CAD build for the part. Positions are in the model's coordinates, mm. Face numbers are marked on the shaded views. Give positions to 0.01 mm unless a question says otherwise; leave off trailing zeros. Loops run counter-clockwise (first coordinate to the right, second up) from the corner with the lowest first, then second, coordinate; pieces in that order, holes last.
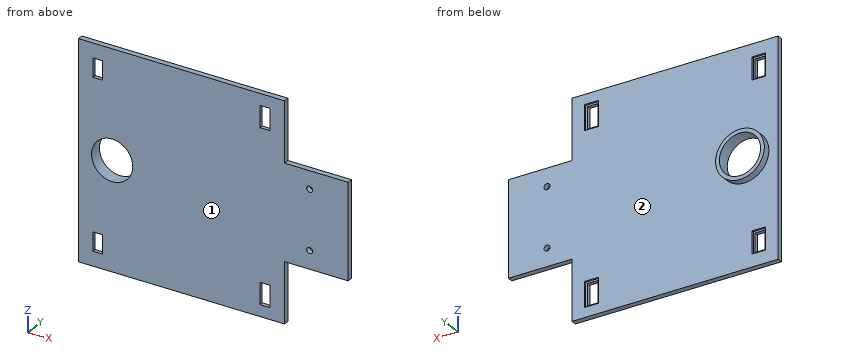
Autodesk Inventor part; units mm, degrees
ref_plane "YZ Plane" through (0, 0, 0) normal (1, 0, 0) x (0, 1, 0)
ref_plane "XZ Plane" through (0, 0, 0) normal (0, 1, 0) x (-1, 0, 0)
ref_plane "XY Plane" through (0, 0, 0) normal (0, 0, 1) x (1, 0, 0)
sketch "Boceto1" plane through (0, 0, 0) normal (0, 1, 0) x (-1, 0, 0)
  line L0 (25.35, 26.5) -> (0, 26.5)
  line L1 (0, 26.5) -> (0, -26.5)
  line L2 (0, -26.5) -> (25.35, -26.5)
  line L3 (-8.9327, 0) -> (109.0416, 0) construction
  line L4 (25.35, 60) -> (150, 60)
  line L5 (150, 60) -> (150, -60)
  line L6 (150, -60) -> (25.35, -60)
  line L7 (25.35, -60) -> (25.35, -26.5)
  line L8 (25.35, 26.5) -> (25.35, 60)
  circle A0 centre (21.45, 16.5) radius 1.65
  circle A1 centre (21.45, -16.5) radius 1.65
  point P0 (0, 0)
  point P1 (0, 0)
  dimension "d1" = 53
  dimension "d2" = 120
  dimension "d3" = 124.65
  dimension "d4" = 25.35
  dimension "d6" = 33.5
  dimension "d8" = 3.3
  dimension "d9" = 16.5
  dimension "d10" = 3.9
extrude "Extrusión1" add sketch "Boceto1" along normal blind 3
sketch "Boceto2" plane through (0, 3, 0) normal (0, 1, 0) x (1, 0, 0)
  line L0 (-150, 60) -> (-150, -60)
  line L1 (-25.35, 60) -> (-150, 60)
  line L2 (-150, -60) -> (-25.35, -60)
  line L3 (-25.35, -60) -> (-25.35, 60)
  line L4 (-25.35, 60) -> (-150, 60)
  line L5 (-150, 60) -> (-150, -60)
  line L6 (-30.35, -55) -> (-145, -55)
  line L7 (-145, -55) -> (-145, 55)
  line L8 (-145, 55) -> (-30.35, 55)
  line L9 (-30.35, 55) -> (-30.35, -55)
  circle A0 centre (-131.25, 0) radius 11.465
  circle A1 centre (-131.25, 0) radius 13.55
  point P0 (0, 0)
  dimension "d13" = 5
  dimension "d14" = 22.93
  dimension "d15" = 13.75
  dimension "d16" = 27.1
extrude "Extrusión2" cut sketch "Boceto2" against normal through all contours A0
extrude "Extrusión3" add sketch "Boceto2" along normal blind 4 contours A1
sketch "Boceto3" plane through (0, 3, 0) normal (0, 1, 0) x (1, 0, 0)
  line L0 (-25.35, 26.5) -> (-25.35, 60)
  line L1 (-25.35, 60) -> (-35.35, 60)
  line L2 (-35.35, 60) -> (-35.35, 26.5)
  line L3 (-35.35, 26.5) -> (-25.35, 26.5)
  line L4 (-25.35, 26.5) -> (-25.35, 60)
  line L5 (-25.35, -60) -> (-25.35, -26.5)
  line L6 (-25.35, -60) -> (-35.35, -60)
  line L7 (-35.35, -60) -> (-35.35, -26.5)
  line L8 (-35.35, -26.5) -> (-25.35, -26.5)
  line L9 (-25.35, -26.5) -> (-25.35, -60)
  point P0 (-150, 60)
  dimension "d46" = 10
  dimension "d47" = 10
  dimension "d48" = 33.5
  dimension "d49" = 33.5
extrude "Extrusión7" cut sketch "Boceto3" against normal through all
sketch "Boceto4" plane through (0, 3, 0) normal (0, 1, 0) x (1, 0, 0)
  line L0 (-143, 53) -> (-135.55, 53)
  line L1 (-135.55, 53) -> (-135.55, 40.55)
  line L2 (-135.55, 40.55) -> (-143, 40.55)
  line L3 (-143, 40.55) -> (-143, 53)
  line L4 (-136.55, 52) -> (-142, 52)
  line L5 (-142, 52) -> (-142, 41.55)
  line L6 (-142, 41.55) -> (-136.55, 41.55)
  line L7 (-136.55, 41.55) -> (-136.55, 52)
  line L8 (-50.1, 54.55) -> (-42.35, 54.55)
  line L9 (-42.35, 54.55) -> (-42.35, 40.55)
  line L10 (-42.35, 40.55) -> (-50.1, 40.55)
  line L11 (-50.1, 40.55) -> (-50.1, 54.55)
  line L12 (-43.35, 53.55) -> (-49.1, 53.55)
  line L13 (-49.1, 53.55) -> (-49.1, 41.55)
  line L14 (-49.1, 41.55) -> (-43.35, 41.55)
  line L15 (-43.35, 41.55) -> (-43.35, 53.55)
  line L16 (-35.35, 60) -> (-150, 60) construction
  line L17 (-35.35, -26.5) -> (-35.35, -60) construction
  line L18 (-150, 60) -> (-35.35, 60) construction
  line L19 (-35.35, 60) -> (-35.35, -60) construction
  line L20 (-35.35, -60) -> (-150, -60) construction
  line L21 (-150, -60) -> (-150, 60) construction
  line L22 (-147, 57) -> (-38.35, 57) construction
  line L23 (-38.35, 57) -> (-38.35, -57) construction
  line L24 (-38.35, -57) -> (-147, -57) construction
  line L25 (-147, -57) -> (-147, 57) construction
  line L26 (-150, 0) -> (0, 0) construction
  line L27 (-50.1, -40.55) -> (-50.1, -54.55)
  line L28 (-136.55, -41.55) -> (-136.55, -52)
  line L29 (-135.55, -53) -> (-135.55, -40.55)
  line L30 (-136.55, -52) -> (-142, -52)
  line L31 (-142, -52) -> (-142, -41.55)
  line L32 (-142, -41.55) -> (-136.55, -41.55)
  line L33 (-143, -53) -> (-135.55, -53)
  line L34 (-135.55, -40.55) -> (-143, -40.55)
  line L35 (-143, -40.55) -> (-143, -53)
  line L36 (-42.35, -40.55) -> (-50.1, -40.55)
  line L37 (-42.35, -54.55) -> (-42.35, -40.55)
  line L38 (-50.1, -54.55) -> (-42.35, -54.55)
  line L39 (-43.35, -53.55) -> (-49.1, -53.55)
  line L40 (-49.1, -53.55) -> (-49.1, -41.55)
  line L41 (-49.1, -41.55) -> (-43.35, -41.55)
  line L42 (-43.35, -41.55) -> (-43.35, -53.55)
  point P0 (-46.225, 40.55)
  point P1 (-139.275, 40.55)
  point P2 (-46.225, -40.55)
  point P3 (-139.275, -40.55)
  dimension "d52" = 7.45
  dimension "d53" = 12.45
  dimension "d54" = 1
  dimension "d55" = 14
  dimension "d56" = 7.75
  dimension "d57" = 1
  dimension "d59" = 3
  dimension "d60" = 4
  dimension "d61" = 4
  dimension "d62" = 4
extrude "Extrusión8" cut sketch "Boceto4" against normal blind 1
extrude "Extrusión9" cut sketch "Boceto4" against normal through all contours L7 L6 L5 L4 | L15 L14 L13 L12 | L28 L30 L31 L32 | L39 L40 L41 L42
properties part number "Base V.2"
1. Drop flat-ended pins along their axis: pin 1 (2.5 mm diameter, centred on x = -21.45, z = -16.5, fed in from +Y); pin 2 (0.8 mm diameter, centred on y = 2.5, z = 43.5, fed in from +X); pin 3 (4 mm diameter, centred on x = -120.5, z = -9, fed in from +Y); pin 4 (2.5 mm diameter, centred on x = -16, y = 1, fed in from -Z). Give the stop position or say it passes through.
Responses:
pin 1: passes through
pin 2: stops at x = -35.35
pin 3: stops at y = 7
pin 4: stops at z = -26.5
2. Pull direction Y, two halves, no side cores. Call the marked faces 1 and 2: released by +Y, released by -Y, zero draft, split by the parting line, or undercut.
Responses:
face 1: released by -Y
face 2: released by +Y
3. Saw through at B-B, the plane z = -16.5. List the corners of the cut face in (x, y), and give its area (3 significant figures).
Responses:
outline: (-150, 0) - (-23.1, 0) - (-23.1, 3) - (-150, 3) - close; (-19.8, 0) - (0, 0) - (0, 3) - (-19.8, 3) - close
area: 440 mm2
4. Saw through at D-D, the plane y = 5.25. List the corners of the cut face in (x, z) (3 decimals).
Responses:
outline: circle Ø27.1 at (-131.25, 0); hole circle Ø22.93 at (-131.25, 0)
5. Saw through at C-C, the plane x = -131.25. List the corners of the cut face in (y, z) (3 decimals).
Responses:
outline: (0, -60) - (3, -60) - (3, -13.55) - (7, -13.55) - (7, -11.465) - (0, -11.465) - close; (0, 11.465) - (7, 11.465) - (7, 13.55) - (3, 13.55) - (3, 60) - (0, 60) - close
6. Probe line 1 along Z through (x, y) = (-21.45, 2.05); line 2 along Z through (x, y) = (-131.25, 2.75) (3 decimals); line 3 along Y through (x, z) = (-107, 16.5). List the from-to ranges inside material, lowest first.
Responses:
line 1: z = -26.5 to -18.15, -14.85 to 14.85, 18.15 to 26.5
line 2: z = -60 to -11.465, 11.465 to 60
line 3: y = 0 to 3
7. Saw through at A-A, the plane z = 45. List the corners of the cut face in (x, y).
Responses:
outline: (-150, 0) - (-142, 0) - (-142, 2) - (-143, 2) - (-143, 3) - (-150, 3) - close; (-136.55, 0) - (-49.1, 0) - (-49.1, 2) - (-50.1, 2) - (-50.1, 3) - (-135.55, 3) - (-135.55, 2) - (-136.55, 2) - close; (-43.35, 0) - (-35.35, 0) - (-35.35, 3) - (-42.35, 3) - (-42.35, 2) - (-43.35, 2) - close
